Here's how the part is built. I have some questions about the finished solid (model axes, mm). Face numbers are marked on the shaded views. A direction names the side the tool comes from. Coordinates: 2 decimals unless noted, no trailing zeros. Order: outer loops, then holes, each group sorted by start corner. A loop starts at its lowest first (then second) coordinate and runs counter-clockwise, first axis right, second up. Notation, with made-up numbers: (32, -30) -> (51, -30) arc R14 cw to (51, -25) -> close; hole circle Ø2 at (38.5, -24.5). An arc over 180 degrees is marked (long way). One line per item, written item: value. Start each with the question number.
```python
from build123d import *

# Parameters (mm, degrees)
F_0000_CYLINDER_SKETCH_R     = 5.5
F_0000_CYLINDER_DEPTH        = 28.5
F_0002_CYLINDER_SKETCH_R     = 2.2
F_0002_CYLINDER_DEPTH        = 24.5
F_0005_CYLINDER_SKETCH_R     = 2
F_0005_CYLINDER_DEPTH        = 6
F_0008_CYLINDER_SKETCH_R     = 4
F_0008_CYLINDER_DEPTH        = 6
F_0008_CYLINDER_ROTATE_ANGLE = 90
F_0010_CYLINDER_SKETCH_R     = 1.6
F_0010_CYLINDER_DEPTH        = 8
F_0010_CYLINDER_ROTATE_ANGLE = 90


with BuildPart() as part:
    # 0000_cylinder_Sketch → 0000_cylinder (new body)
    with BuildSketch(Plane.XY):
        with Locations(Location((0, 0, 0), (0, 0, 180))):
            Circle(F_0000_CYLINDER_SKETCH_R)
    extrude(amount=F_0000_CYLINDER_DEPTH)


with BuildPart() as part_1:
    # 0000_cylinder_Translate: moved
    add(part.part.moved(Location((0, 0, 7))))


with BuildPart() as body_2:
    # 0002_cylinder_Sketch → 0002_cylinder (new body)
    with BuildSketch(Plane.XY):
        Circle(F_0002_CYLINDER_SKETCH_R)
    extrude(amount=F_0002_CYLINDER_DEPTH)


with BuildPart() as body_2_1:
    # 0002_cylinder_Translate: moved
    add(body_2.part.moved(Location((0, 0, 12))))


with BuildPart() as part_2:
    add(part_1.part)

    # 0004_sub: cut body 2
    add(body_2_1.part, mode=Mode.SUBTRACT)


with BuildPart() as body_2_2:
    # 0005_cylinder_Sketch → 0005_cylinder (new body)
    with BuildSketch(Plane.XY):
        Circle(F_0005_CYLINDER_SKETCH_R)
    extrude(amount=F_0005_CYLINDER_DEPTH)


with BuildPart() as body_2_2_1:
    # 0005_cylinder_Translate: moved
    add(body_2_2.part.moved(Location((0, 0, 3))))


with BuildPart() as part_3:
    add(part_2.part)

    # 0007_add: union body 2 2
    add(body_2_2_1.part)


with BuildPart() as body_2_3:
    # 0008_cylinder_Sketch → 0008_cylinder (new body)
    with BuildSketch(Plane.XY):
        Circle(F_0008_CYLINDER_SKETCH_R)
    extrude(amount=F_0008_CYLINDER_DEPTH)


with BuildPart() as body_2_3_1:
    # 0008_cylinder_Rotate: moved
    add(body_2_3.part.rotate(Axis((0, 0, 0), (0, 1, 0)), F_0008_CYLINDER_ROTATE_ANGLE))


with BuildPart() as body_2_3_2:
    # 0008_cylinder_Translate: moved
    add(body_2_3_1.part.moved(Location((-3, 0, 0))))


with BuildPart() as part_4:
    add(part_3.part)

    # 0009_add: union body 2 3
    add(body_2_3_2.part)


with BuildPart() as body_2_4:
    # 0010_cylinder_Sketch → 0010_cylinder (new body)
    with BuildSketch(Plane.XY):
        Circle(F_0010_CYLINDER_SKETCH_R)
    extrude(amount=F_0010_CYLINDER_DEPTH)


with BuildPart() as body_2_4_1:
    # 0010_cylinder_Rotate: moved
    add(body_2_4.part.rotate(Axis((0, 0, 0), (0, 1, 0)), F_0010_CYLINDER_ROTATE_ANGLE))


with BuildPart() as body_2_4_2:
    # 0010_cylinder_Translate: moved
    add(body_2_4_1.part.moved(Location((-4, 0, 0))))


with BuildPart() as part_5:
    add(part_4.part)

    # 0011_sub: cut body 2 4
    add(body_2_4_2.part, mode=Mode.SUBTRACT)


solid = part_5.part
```
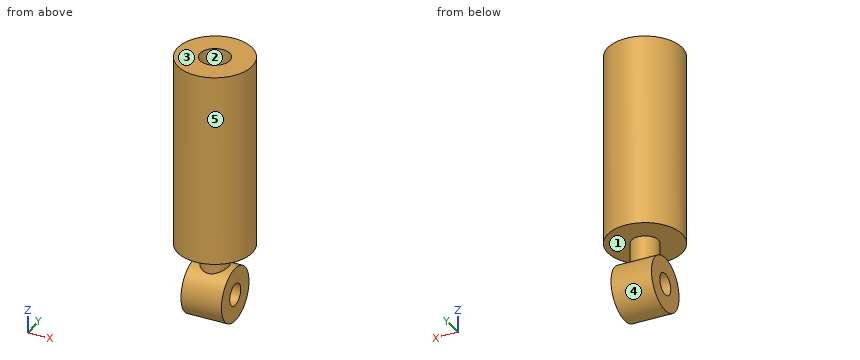
Q1. For P1, Ø4, axis at y = 0.5, z = 1.5, coming from the -X side; P2, Ø1.9, axis at y = 0, z = 0, coming from the -X side; P3, Ø2, axis at y = 3, z = 10, coming from the -X side; P4, Ø6.5, axis at y = 0, z = 1, coming from the +X side, each with a flat end and sliding along its axis, tell me the tip position at first contact or that it passes through.
Q2. Imagine slicing it at B-B (x = 0). Write out the boundary of the cut face in (y, z), plus the area to 3 significant figures.
Q3. If we mould it in two halves opening along Z, with no side actions, what happens to the marked faces 3, 4 and 5? For each: +Z half, -Z half, draft (parallel to the pull), parting line (faces both ways), or undercut.
Q4. Imagine slicing it at D-D (z = 24). Write out the boundary of the cut face in (x, y), plus the area to 3 significant figures.
Q5. Imagine slicing it at A-A (z = 0). Write out the boundary of the cut face in (x, y), plus the area to 3 significant figures.
Q6. Imagine slicing it at C-C (y = 0). Write out the boundary of the cut face in (x, z), plus the area to 3 significant figures.
Q7. I need wall thicknesses on line 1 (Z direction, x = -2.5, y = 0); line 2 (Y direction, x = 0, z = 28); line 3 (Y direction, x = -0.7, z = 0). Which ranges of each line are inside material? Lowest first, please.
Q8. For the marked faces 1 and 2, which set-ups out of +Z, -Z, +X, -X, +Y, -Y let a thin tool reach every point of the face, with its end or its side?
Completed:
1. P1: stops at x = -3
1. P2: passes through
1. P3: stops at x = -5.12
1. P4: stops at x = 3
2. outline: (-5.5, 7) -> (-2, 7) -> (-2, 3.46) arc R4 ccw (long way) to (2, 3.46) -> (2, 7) -> (5.5, 7) -> (5.5, 35.5) -> (2.2, 35.5) -> (2.2, 12) -> (-2.2, 12) -> (-2.2, 35.5) -> (-5.5, 35.5) -> close; hole circle Ø3.2 at (0, 0)
2. area: 265 mm2
3. face 3: +Z half
3. face 4: undercut
3. face 5: draft
4. outline: circle Ø11 at (0, 0); hole circle Ø4.4 at (0, 0)
4. area: 79.8 mm2
5. outline: (-3, -4) -> (3, -4) -> (3, -1.6) -> (-3, -1.6) -> close; (-3, 1.6) -> (3, 1.6) -> (3, 4) -> (-3, 4) -> close
5. area: 28.8 mm2
6. outline: (-5.5, 7) -> (-2, 7) -> (-2, 4) -> (-3, 4) -> (-3, 1.6) -> (3, 1.6) -> (3, 4) -> (2, 4) -> (2, 7) -> (5.5, 7) -> (5.5, 35.5) -> (2.2, 35.5) -> (2.2, 12) -> (-2.2, 12) -> (-2.2, 35.5) -> (-5.5, 35.5) -> close; (-3, -4) -> (3, -4) -> (3, -1.6) -> (-3, -1.6) -> close
6. area: 251 mm2
7. line 1: z = -4 to -1.6, 1.6 to 4, 7 to 35.5
7. line 2: y = -5.5 to -2.2, 2.2 to 5.5
7. line 3: y = -4 to -1.6, 1.6 to 4
8. face 1: none
8. face 2: +Z
